from build123d import *
from build123d import SkipClean  # not in build123d's __all__

# Parameters (mm, degrees)
F0_W      = 70
F0_H      = 60
F8_DEPTH  = 20
F1_W      = 10
F1_H      = 60
F9_DEPTH  = 60
F10_DEPTH = 25
F3_DEPTH  = 40
F4_DEPTH  = 60
F11_DEPTH = 109.889773652
F6_W      = 20
F6_H      = 60
F12_DEPTH = 60
F14_DEPTH = 25
F7_DEPTH  = 20


with BuildPart() as f8:
    # F0 (on Front) → F8 (new body)
    with BuildSketch(Plane.XZ):
        with Locations((-39.945468749, 30)):
            Rectangle(F0_W, F0_H)
    extrude(amount=F8_DEPTH)

    # F1 (on face) → F9 (join)
    with BuildSketch(Plane.XZ.offset(20)):
        with Locations((-9.945468749, 30)):
            Rectangle(F1_W, F1_H)
    extrude(amount=F9_DEPTH)

    # F2 (on face) → F10 (join)
    with BuildSketch(Plane(origin=(-14.945468749, 0, 0), x_dir=(0, -1, 0), z_dir=(-1, 0, 0))):
        with BuildLine():
            Line((55.5051025722, 35), (50.4196010845, 35))
            ThreePointArc((50.4196010845, 35), (50, 30), (50.4196010845, 25))
            Line((50.4196010845, 25), (55.5051025722, 25))
            ThreePointArc((55.5051025722, 25), (55, 30), (55.5051025722, 35))
        make_face()
        with BuildLine():
            Line((55.5051025722, 25), (50.4196010845, 25))
            ThreePointArc((50.4196010845, 25), (60.635083269, 7.0871215252), (80, 0))
            Line((80, 0), (80, 5))
            ThreePointArc((80, 5), (64.1886116992, 10.635083269), (55.5051025722, 25))
        make_face()
        with BuildLine():
            ThreePointArc((80, 60), (60.635083269, 52.9128784748), (50.4196010845, 35))
            Line((50.4196010845, 35), (55.5051025722, 35))
            ThreePointArc((55.5051025722, 35), (64.1886116992, 49.364916731), (80, 55))
            Line((80, 55), (80, 60))
        make_face()
        with BuildLine():
            ThreePointArc((110, 30), (101.2132034356, 51.2132034356), (80, 60))
            Line((80, 60), (80, 55))
            ThreePointArc((80, 55), (97.6776695297, 47.6776695297), (105, 30))
            ThreePointArc((105, 30), (97.6776695297, 12.3223304703), (80, 5))
            Line((80, 5), (80, 0))
            ThreePointArc((80, 0), (101.2132034356, 8.7867965644), (110, 30))
        make_face()
    extrude(amount=F10_DEPTH)

    # F3 (add): a face of the model
    f3_faces = [f8.faces().sort_by_distance(p)[0] for p in [
        (-39.945468749, -80, 4.1514718626),
    ]]
    extrude(f3_faces, amount=-F3_DEPTH)

    # F2 (on face) → F4 (join)
    with BuildSketch(Plane(origin=(-14.945468749, 0, 0), x_dir=(0, -1, 0), z_dir=(-1, 0, 0))):
        with BuildLine():
            Line((50.4196010845, 35), (20, 35))
            Line((20, 35), (20, 25))
            Line((20, 25), (50.4196010845, 25))
            ThreePointArc((50.4196010845, 25), (50, 30), (50.4196010845, 35))
        make_face()
    extrude(amount=F4_DEPTH)

    # F5 (on face) → F11 (cut)
    with BuildSketch(Plane(origin=(0, 0, 25), x_dir=(1, 0, 0), z_dir=(0, 0, -1))):
        Polygon((-74.945468749, 50.4196010845), (-74.945468749, 20), (-39.945468749, 50.4196010845), align=None)
    extrude(amount=-F11_DEPTH, mode=Mode.SUBTRACT)

    # F6 (on face) → F12 (join)
    with BuildSketch(Plane.XZ):
        with Locations((-64.945468749, 30)):
            Rectangle(F6_W, F6_H)
    extrude(amount=-F12_DEPTH)

    # F13 (on face) → F14 (cut)
    with BuildSketch(Plane(origin=(-74.945468749, 0, 0), x_dir=(0, -1, 0), z_dir=(-1, 0, 0))):
        with BuildLine():
            Line((0, 60), (-20, 60))
            ThreePointArc((-20, 60), (-17.0710678119, 52.9289321881), (-10, 50))
            ThreePointArc((-10, 50), (-2.9289321881, 52.9289321881), (0, 60))
        make_face()
        with BuildLine():
            Line((-10, 10), (-60, 10))
            Line((-60, 10), (-60, 0))
            Line((-60, 0), (-20, 0))
            ThreePointArc((-20, 0), (-17.0710678119, 7.0710678119), (-10, 10))
        make_face()
        with BuildLine():
            ThreePointArc((0, 0), (-2.9289321881, 7.0710678119), (-10, 10))
            ThreePointArc((-10, 10), (-17.0710678119, 7.0710678119), (-20, 0))
            Line((-20, 0), (0, 0))
        make_face()
        with BuildLine():
            ThreePointArc((-10, 50), (-17.0710678119, 52.9289321881), (-20, 60))
            Line((-20, 60), (-60, 60))
            Line((-60, 60), (-60, 50))
            Line((-60, 50), (-10, 50))
        make_face()
        with BuildLine():
            ThreePointArc((-52.5, 30), (-54.6966991411, 35.3033008589), (-60, 37.5))
            Line((-60, 37.5), (-60, 22.5))
            ThreePointArc((-60, 22.5), (-54.6966991411, 24.6966991411), (-52.5, 30))
        make_face()
    extrude(amount=-F14_DEPTH, mode=Mode.SUBTRACT)

    # F13 (on face) → F7 (join)
    with BuildSketch(Plane(origin=(-74.945468749, 0, 0), x_dir=(0, -1, 0), z_dir=(-1, 0, 0))):
        with BuildLine():
            Line((-60, 37.5), (-60, 50))
            ThreePointArc((-60, 50), (-80, 30), (-60, 10))
            Line((-60, 10), (-60, 22.5))
            ThreePointArc((-60, 22.5), (-67.5, 30), (-60, 37.5))
        make_face()
        with BuildLine():
            ThreePointArc((-40, 30), (-45.8578643763, 44.1421356237), (-60, 50))
            Line((-60, 50), (-60, 37.5))
            ThreePointArc((-60, 37.5), (-54.6966991411, 35.3033008589), (-52.5, 30))
            ThreePointArc((-52.5, 30), (-54.6966991411, 24.6966991411), (-60, 22.5))
            Line((-60, 22.5), (-60, 10))
            ThreePointArc((-60, 10), (-45.8578643763, 15.8578643763), (-40, 30))
        make_face()
    with SkipClean():  # cleaning this boolean's faces spoils the solid; the shape is the same uncleaned
        extrude(amount=-F7_DEPTH)


solid = f8.part
Design review of the part built by this model. Coordinates are the model's own, in mm. A direction names the side the tool comes from. Coordinates: 2 decimals unless noted, no trailing zeros. Loops run counter-clockwise (first coordinate to the right, second up) from the corner with the lowest first, then second, coordinate; pieces in that order, holes last. Notation, with made-up numbers: (-35, 62.25) -> (-25, 62.25) arc R26 ccw to (-25, 79.25) -> close; hole circle Ø4 at (30, 3). An arc over 180 degrees is marked (long way). Use a Markdown table: item, result. Add a question column.
Item 1: We need section D-D, the plane x = -61. Write out the cut boundary in (y, z).
Item 2: We need section C-C, the plane y = -97. Write out the cut boundary in (x, z).
Item 3: The part is to be moulded in two halves that separate along Y. For faces 1 (the flat face through (-4.945, -70, 30)), 2 (the flat face through (-65, 35, 50)), 3 (the flat face through (-57.69, -34.997, 29.93)), 4 (the flat face through (-30, 0, 30)), say which applies: +Y half, -Y half, draft (parallel to the pull), parting line (faces both ways), or undercut.
Item 4: We need section B-B, the plane x = -32. Write out the cut boundary in (y, z), and give its area (3 significant figures).
Item 5: Wall thickness on L1, parallel to Z at x = -31.75, y = -80; L2, parallel to Y at x = -31, z = 37.5; L3, parallel to Z at x = -68.75, y = 60: over which ranges is each line inside the solid? List them lowest first. Write a range as from..to.
Item 6: Machinability: for faces 5 (the flat face through (-14.945, -70, 30)), 6 (the flat face through (-45, -20, 48)), 7 (the flat face through (-45, -20, 13)), 8 (the flat face through (-10, -80, 30)), which of the approach directions +Z, -Z, +X, -X, +Y, -Y give a long, thin tool a straight path to every point of the face, cutting with its end or side? Answer none if there is none.
Item 7: Clearance check with flat-ended pins moving along their axes: P1, Ø1, axis at y = 26, z = 37, coming from the +X side; P2, Ø12.5, axis at y = -46, z = 12, coming from the -X side; P3, Ø24.5, axis at x = -58.5, y = -37, coming from the +Z side. State where each tip first meets the part, or that it passes through.
Item 8: We need section A-A, the plane z = 30. Write out the cut boundary in (x, y).
Numbers:
| question | item | result |
|---|---|---|
| 1 | outline | (-32.12, 25) -> (-20, 25) -> (-20, 0) -> (0, 0) arc R10 cw to (10, 10) -> (60, 10) arc R20 ccw to (60, 50) -> (10, 50) arc R10 cw to (0, 60) -> (-20, 60) -> (-20, 35) -> (-32.12, 35) -> close; hole circle Ø15 at (60, 30) |
| 2 | outline | (-39.95, 5.28) -> (0.05, 5.28) -> (0.05, 11.67) -> (-39.95, 11.67) -> close; (-39.95, 48.33) -> (0.05, 48.33) -> (0.05, 54.72) -> (-39.95, 54.72) -> close |
| 3 | face 1 | undercut |
| 3 | face 2 | draft |
| 3 | face 3 | -Y half |
| 3 | face 4 | +Y half |
| 4 | outline | (-50.42, 25) -> (-20, 25) -> (-20, 0) -> (0, 0) -> (0, 60) -> (-20, 60) -> (-20, 35) -> (-50.42, 35) arc R30 ccw (long way) to start; hole circle Ø50 at (-80, 30) |
| 4 | area | 2,370 mm^2 |
| 5 | L1 | z = 0..5, 55..60 |
| 5 | L2 | y = -109.05..-103.85, -56.15..-50.95, -20..0 |
| 5 | L3 | z = 10..22.5, 37.5..50 |
| 6 | face 5 | -X |
| 6 | face 6 | +Z, -X |
| 6 | face 7 | -Z, -X |
| 6 | face 8 | +X, -X |
| 7 | P1 | stops at x = -54.95 |
| 7 | P2 | stops at x = -14.95 |
| 7 | P3 | stops at z = 35 |
| 8 | outline | (-74.95, -20) -> (-40.43, -50) -> (-39.95, -50) -> (-39.95, -55) -> (-14.95, -55) -> (-14.95, -80) -> (-4.95, -80) -> (-4.95, -55) -> (0.05, -55) -> (0.05, -50) -> (-4.95, -50) -> (-4.95, 0) -> (-54.95, 0) -> (-54.95, 52.5) -> (-74.95, 52.5) -> close; (-74.95, 67.5) -> (-54.95, 67.5) -> (-54.95, 80) -> (-74.95, 80) -> close; (-39.95, -110) -> (0.05, -110) -> (0.05, -105) -> (-39.95, -105) -> close |
